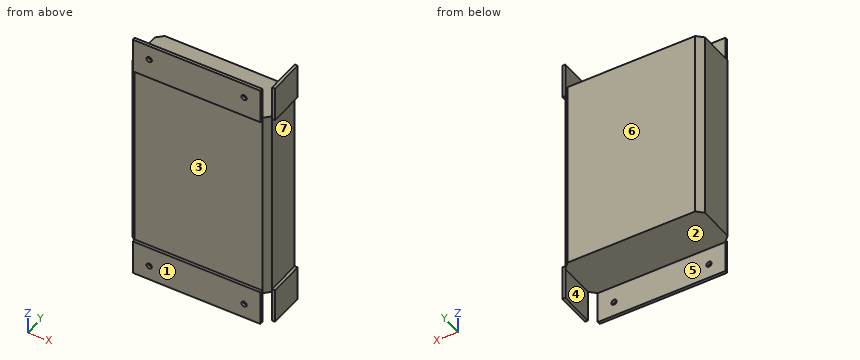
from build123d import *

# Parameters (mm, degrees)
SKETCH1_W                = 83.4
SKETCH1_H                = 28.65
BOSS_EXTRUDE1_DEPTH      = 115.25
CHAMFER1_SIZE            = 3.6
BOSS_EXTRUDE2_DEPTH      = 19
BOSS_EXTRUDE2_DEPTH_BACK = 1.75
SKETCH2_W                = 1.75
SKETCH2_H                = 21.45
SKETCH2_W_2              = 76.2
SKETCH2_H_2              = 1.75
BOSS_EXTRUDE4_DEPTH      = 1.75
BOSS_EXTRUDE4_DEPTH_BACK = 19
BOSS_EXTRUDE4_START      = -115.25
SKETCH2_2_W              = 1.75
SKETCH2_2_H              = 21.45
SKETCH2_2_W_2            = 76.2
SKETCH2_2_H_2            = 1.75
SKETCH3_R                = 1.6
CUT_EXTRUDE1_DEPTH       = 144.985372521


with BuildPart() as part:
    # Sketch1 → Boss-Extrude1 (new body)
    with BuildSketch(Plane.XY):
        Rectangle(SKETCH1_W, SKETCH1_H)
    extrude(amount=BOSS_EXTRUDE1_DEPTH)

    # Chamfer1
    chamfer1_edges = [part.edges().sort_by_distance(p)[0] for p in [
        (41.7, -14.325, 57.625),
        (-41.7, -14.325, 57.625),
        (-41.7, 14.325, 57.625),
        (41.7, 14.325, 57.625),
    ]]
    chamfer(chamfer1_edges, length=CHAMFER1_SIZE)

    # Sketch2 → Boss-Extrude2 (add, two sides: drawn at the far end of the back side and taken through both)
    with BuildSketch(Plane.XY.offset(115.25).offset(-BOSS_EXTRUDE2_DEPTH_BACK)):
        with Locations((42.575, 0)):
            Rectangle(SKETCH2_W, SKETCH2_H)
        with Locations((0, -15.2)):
            Rectangle(SKETCH2_W_2, SKETCH2_H_2)
    extrude(amount=BOSS_EXTRUDE2_DEPTH + BOSS_EXTRUDE2_DEPTH_BACK)

    # Sketch2_2 → Boss-Extrude4 (add, two sides: drawn at the far end of the back side and taken through both)
    with BuildSketch(Plane.XY.offset(115.25).offset(BOSS_EXTRUDE4_START - BOSS_EXTRUDE4_DEPTH_BACK)):
        with Locations((42.575, 0)):
            Rectangle(SKETCH2_2_W, SKETCH2_2_H)
        with Locations((0, -15.2)):
            Rectangle(SKETCH2_2_W_2, SKETCH2_2_H_2)
    extrude(amount=BOSS_EXTRUDE4_DEPTH + BOSS_EXTRUDE4_DEPTH_BACK)

    # Sketch3 → Cut-Extrude1 (cut, through all)
    with BuildSketch(Plane(origin=(0, -14.325, 0), x_dir=(1, 0, 0), z_dir=(0, 1, 0))):
        with Locations(Location((-28.321, 10.193, 0), (0, 0, 180))):
            Circle(SKETCH3_R)
        with Locations(Location((28.321, 10.193, 0), (0, 0, 180))):
            Circle(SKETCH3_R)
        with Locations(Location((28.321, -125.443, 0), (0, 0, 180))):
            Circle(SKETCH3_R)
        with Locations(Location((-28.321, -125.443, 0), (0, 0, 180))):
            Circle(SKETCH3_R)
    extrude(amount=-CUT_EXTRUDE1_DEPTH, mode=Mode.SUBTRACT)


solid = part.part
Part model, mm, in its own coordinate system. Face numbers are marked on the shaded views. A direction names the side the tool comes from. Coordinates: 2 decimals unless noted, no trailing zeros. Write each loop counter-clockwise with the first axis right and the second up, starting at its lowest first coordinate (ties: lowest second). Pieces come first, ordered by that corner, then holes. Notation, with made-up numbers: M -34,52 L 21,52 A23 ccw 21,91 Z; hole C 8.25,19.5 d1. An arc over 180 degrees is marked long. Return JSON: item names as keys, results as strings.
1. Flat gauge pins, fed straight in: pin 1 Ø0.5 at (x, z) = (42.5, 128) entering from -Y (3 decimals); pin 2 Ø9.5 at (x, z) = (-17.5, 123.5) entering from +Y (3 decimals); pin 3 Ø1.4 at (x, z) = (42.5, -10) entering from +Y (3 decimals); pin 4 Ø2.5 at (x, z) = (28.321, -10.193) entering from -Y. Where does each tip first touch, or does it go through?
Determined:
{"pin 1": "y = -10.725", "pin 2": "y = -14.325", "pin 3": "y = 10.725", "pin 4": "through"}
2. Saw through at B-B, the plane x = -32. Write the cut outline in (y, z) (3 decimals), then the cut area to 3 significant figures.
Determined:
{"outline": "M -16.075,-19 L -14.325,-19 L -14.325,0 L 14.325,0 L 14.325,115.25 L -14.325,115.25 L -14.325,134.25 L -16.075,134.25 L -16.075,113.5 L -14.325,113.5 L -14.325,1.75 L -16.075,1.75 Z", "area": "3,370 mm²"}
3. Saw through at A-A, the plane z = 13. Write the cut outline in (x, y) (3 decimals), then the cut area to 3 significant figures.
Determined:
{"outline": "M -41.7,-10.725 L -38.1,-14.325 L 38.1,-14.325 L 41.7,-10.725 L 41.7,10.725 L 38.1,14.325 L -38.1,14.325 L -41.7,10.725 Z", "area": "2,360 mm²"}
4. Pull direction Z, two halves, no side cores. Call the marked faces 1, 2 and 3: pulls with the +Z half, pulls with the -Z half, needs draft (parallel to the pull), parting line crosses it, or undercut.
Determined:
{"face 1": "needs draft", "face 2": "pulls with the -Z half", "face 3": "undercut"}
5. 3-axis set-ups, long thin cutter, end or side, ignore diameter. For the marked faces 4, 5, 6 and 7: which of +Z, -Z, +X, -X, +Y, -Y reach the whole face in a straight line?
Determined:
{"face 4": "-Z, -X, +Y, -Y", "face 5": "-Z, +X, -X, +Y", "face 6": "+Z, -Z, +X, -X, +Y", "face 7": "+X, +Y, -Y"}
6. Probe L1, parallel to Z at x = 37, y = -5; L2, parallel to Y at x = -23, z = 14 (3 decimals); L3, parallel to Y at x = 20.5, z = 116 (3 decimals). List the from-to ranges inside material, lowest first.
Determined:
{"L1": "0 to 115.25", "L2": "-14.325 to 14.325", "L3": "-16.075 to -14.325"}
7. Saw through at C-C, the plane y = 7. Write the cut outline in (x, z).
Determined:
{"outline": "M -41.7,0 L 41.7,0 L 41.7,-19 L 43.45,-19 L 43.45,1.75 L 41.7,1.75 L 41.7,113.5 L 43.45,113.5 L 43.45,134.25 L 41.7,134.25 L 41.7,115.25 L -41.7,115.25 Z"}
